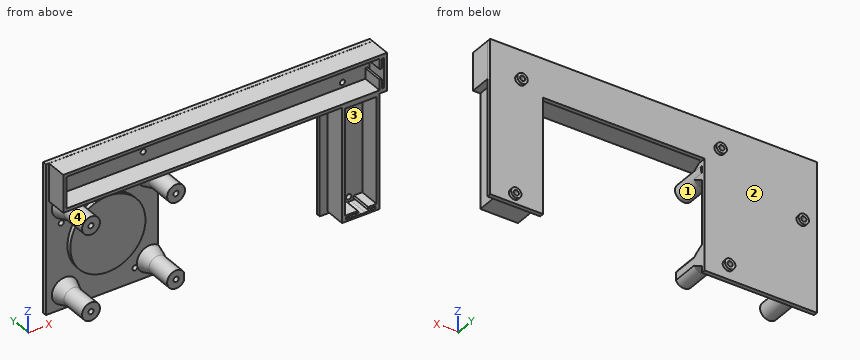
from build123d import *

# Parameters (mm, degrees)
SKETCH1_W                 = 25.299499494
SKETCH1_H                 = 55.159009877
SKETCH1_R                 = 1.241657959
SKETCH1_R_2               = 1.244649804
SKETCH1_R_3               = 1.243452392
SKETCH1_W_2               = 53.713568487
SKETCH1_H_2               = 52.951897156
SKETCH1_R_4               = 1.244762628
SKETCH1_R_5               = 1.240228495
BOSS_EXTRUDE1_DEPTH       = 2
SKETCH2_R                 = 2.521764251
SKETCH2_R_2               = 1.240228495
SKETCH2_R_3               = 2.471513498
SKETCH2_R_4               = 1.244762628
SKETCH2_R_5               = 2.485581318
SKETCH2_R_6               = 1.244649804
SKETCH2_R_7               = 2.50000008
SKETCH2_R_8               = 1.232345201
SKETCH2_R_9               = 2.472424153
SKETCH2_R_10              = 1.241657959
BOSS_EXTRUDE2_DEPTH       = 1.5
BOSS_EXTRUDE3_OUTLINE_R   = 4.264975471
BOSS_EXTRUDE3_OUTLINE_R_2 = 1.25
BOSS_EXTRUDE3_OUTLINE_R_3 = 4.293360572
BOSS_EXTRUDE3_DEPTH       = 18.2
BOSS_EXTRUDE4_OUTLINE_W   = 148.81215391
BOSS_EXTRUDE4_OUTLINE_H   = 14.000040224
BOSS_EXTRUDE4_DEPTH       = 10
SKETCH7_W                 = 18.030681689
SKETCH7_H                 = 1.47954917
BOSS_EXTRUDE5_DEPTH       = 10
SKETCH8_R                 = 2.5
SKETCH8_W                 = 14.030681689
SKETCH8_H                 = 1
CUT_EXTRUDE1_DEPTH        = 16.42
SKETCH9_W                 = 2
SKETCH9_H                 = 18.000040224
BOSS_EXTRUDE6_DEPTH       = 10
SKETCH10_W                = 1
SKETCH10_H                = 14.000040224
SKETCH10_W_2              = 1.5
SKETCH10_H_2              = 5
CUT_EXTRUDE2_DEPTH        = 10
CHAMFER1_SIZE             = 2
CHAMFER1_SIZE_2           = 5.494954839
SKETCH12_W                = 15.030681689
SKETCH12_H                = 50.706334577
SKETCH12_W_2              = 14.030681689
SKETCH12_H_2              = 49.706334577
SKETCH12_W_3              = 149.81215391
SKETCH12_H_3              = 15.000040224
SKETCH12_W_4              = 148.81215391
SKETCH12_H_4              = 14.000040224
CUT_EXTRUDE3_DEPTH        = 16.42
SKETCH13_R                = 17.983803221
BOSS_EXTRUDE7_DEPTH       = 2


# Read off the part's stored shape, not the designer's step: Boss-Extrude3, Boss-Extrude4
with BuildPart() as part:
    # Sketch1 → Boss-Extrude1 (new body)
    # profile 1 of 3: a face of its own
    with BuildSketch(Plane(origin=(0, 0, 0), x_dir=(1, 0, 0), z_dir=(0, 1, 0))):
        with Locations((-12.099843009, -21.166171701)):
            Rectangle(SKETCH1_W, SKETCH1_H)
        with Locations(Location((-10.884458073, 2.271979315, 0), (0, 0, 270))):
            Circle(SKETCH1_R, mode=Mode.SUBTRACT)
    # profile 2 of 3: a face of its own
    with BuildSketch(Plane(origin=(0, 0, 0), x_dir=(1, 0, 0), z_dir=(0, 1, 0))):
        Polygon((0.549906738, -67.187297417), (0.549906738, -48.745676639), (-24.749592756, -48.745676639), (-102.011751733, -48.745676639), (-155.72532022, -48.745676639), (-155.72532022, -67.187297417), align=None)
        with Locations(Location((-109.139310681, -55.741320352, 0), (0, 0, 270))):
            Circle(SKETCH1_R_2, mode=Mode.SUBTRACT)
        with Locations(Location((-13.892677204, -53.014877456, 0), (0, 0, 270))):
            Circle(SKETCH1_R_3, mode=Mode.SUBTRACT)
    # profile 3 of 3: a face of its own
    with BuildSketch(Plane(origin=(0, 0, 0), x_dir=(1, 0, 0), z_dir=(0, 1, 0))):
        with Locations((-128.868535977, -22.269728061)):
            Rectangle(SKETCH1_W_2, SKETCH1_H_2)
        with Locations(Location((-148.388511799, -36.727074265, 0), (0, 0, 270))):
            Circle(SKETCH1_R_4, mode=Mode.SUBTRACT)
        with Locations(Location((-113.148248588, -2.237044718, 0), (0, 0, 270))):
            Circle(SKETCH1_R_5, mode=Mode.SUBTRACT)
    extrude(amount=BOSS_EXTRUDE1_DEPTH)

    # Sketch2 → Boss-Extrude2 (add)
    # profile 1 of 5: a face of its own
    with BuildSketch(Plane(origin=(0, 2, 0), x_dir=(1, 0, 0), z_dir=(0, 1, 0))):
        with Locations(Location((-113.148248588, -2.237044718, 0), (0, 0, 270))):
            Circle(SKETCH2_R)
        with Locations(Location((-113.148248588, -2.237044718, 0), (0, 0, 270))):
            Circle(SKETCH2_R_2, mode=Mode.SUBTRACT)
    # profile 2 of 5: a face of its own
    with BuildSketch(Plane(origin=(0, 2, 0), x_dir=(1, 0, 0), z_dir=(0, 1, 0))):
        with Locations(Location((-148.388511799, -36.727074265, 0), (0, 0, 270))):
            Circle(SKETCH2_R_3)
        with Locations(Location((-148.388511799, -36.727074265, 0), (0, 0, 270))):
            Circle(SKETCH2_R_4, mode=Mode.SUBTRACT)
    # profile 3 of 5: a face of its own
    with BuildSketch(Plane(origin=(0, 2, 0), x_dir=(1, 0, 0), z_dir=(0, 1, 0))):
        with Locations(Location((-109.139310681, -55.741320352, 0), (0, 0, 270))):
            Circle(SKETCH2_R_5)
        with Locations(Location((-109.139310681, -55.741320352, 0), (0, 0, 270))):
            Circle(SKETCH2_R_6, mode=Mode.SUBTRACT)
    # profile 4 of 5: a face of its own
    with BuildSketch(Plane(origin=(0, 2, 0), x_dir=(1, 0, 0), z_dir=(0, 1, 0))):
        with Locations(Location((-13.886720738, -53.00550248, 0), (0, 0, 270))):
            Circle(SKETCH2_R_7)
        with Locations(Location((-13.886720738, -53.00550248, 0), (0, 0, 57.569834669))):
            Circle(SKETCH2_R_8, mode=Mode.SUBTRACT)
    # profile 5 of 5: a face of its own
    with BuildSketch(Plane(origin=(0, 2, 0), x_dir=(1, 0, 0), z_dir=(0, 1, 0))):
        with Locations(Location((-10.884458073, 2.271979315, 0), (0, 0, 270))):
            Circle(SKETCH2_R_9)
        with Locations(Location((-10.884458073, 2.271979315, 0), (0, 0, 270))):
            Circle(SKETCH2_R_10, mode=Mode.SUBTRACT)
    extrude(amount=BOSS_EXTRUDE2_DEPTH)

    # Boss-Extrude3 outline → Boss-Extrude3 (add)
    # profile 1 of 4: a face of its own
    with BuildSketch(Plane.XZ):
        with Locations((-105.874082677, 44.738348581)):
            Circle(BOSS_EXTRUDE3_OUTLINE_R)
        with Locations((-105.874082677, 44.738348581)):
            Circle(BOSS_EXTRUDE3_OUTLINE_R_2, mode=Mode.SUBTRACT)
    # profile 2 of 4: a face of its own
    with BuildSketch(Plane.XZ):
        with BuildLine():
            ThreePointArc((-102.011751733, 5.914823562), (-110.167443249, 4.039898313), (-102.011751733, 2.164973064))
            Line((-102.011751733, 2.164973064), (-102.011751733, 5.914823562))
        make_face()
        with Locations((-105.874082677, 4.039898313)):
            Circle(BOSS_EXTRUDE3_OUTLINE_R_2, mode=Mode.SUBTRACT)
    # profile 3 of 4: a face of its own
    with BuildSketch(Plane.XZ):
        with Locations((-146.574082677, 4.039898313)):
            Circle(BOSS_EXTRUDE3_OUTLINE_R_3)
        with Locations((-146.574082677, 4.039898313)):
            Circle(BOSS_EXTRUDE3_OUTLINE_R_2, mode=Mode.SUBTRACT)
    # profile 4 of 4: a face of its own
    with BuildSketch(Plane.XZ):
        with Locations((-146.574082677, 44.738348581)):
            Circle(BOSS_EXTRUDE3_OUTLINE_R)
        with Locations((-146.574082677, 44.738348581)):
            Circle(BOSS_EXTRUDE3_OUTLINE_R_2, mode=Mode.SUBTRACT)
    extrude(amount=BOSS_EXTRUDE3_DEPTH)

    # Boss-Extrude4 outline → Boss-Extrude4 (add)
    with BuildSketch(Plane.XZ):
        Polygon((-2.890953027, -4.07972047), (-2.890953027, 49.144078772), (-1.415765517, 49.144078772), (-1.415765517, 67.144118996), (-154.227919427, 67.144118996), (-154.227919427, 49.144078772), (-20.921634716, 49.144078772), (-20.921634716, -4.07972047), align=None)
        with BuildLine():
            ThreePointArc((-9.657775138, -2.07972047), (-10.884458073, -3.513637274), (-12.111141008, -2.07972047))
            Line((-12.111141008, -2.07972047), (-18.921634716, -2.07972047))
            Line((-18.921634716, -2.07972047), (-18.921634716, 47.626614107))
            Line((-18.921634716, 47.626614107), (-4.890953027, 47.626614107))
            Line((-4.890953027, 47.626614107), (-4.890953027, -2.07972047))
            Line((-4.890953027, -2.07972047), (-9.657775138, -2.07972047))
        make_face(mode=Mode.SUBTRACT)
        with Locations((-77.821842472, 58.144098884)):
            Rectangle(BOSS_EXTRUDE4_OUTLINE_W, BOSS_EXTRUDE4_OUTLINE_H, mode=Mode.SUBTRACT)
    extrude(amount=BOSS_EXTRUDE4_DEPTH)

    # Sketch7 → Boss-Extrude5 (add)
    with BuildSketch(Plane.XZ):
        with Locations((-11.906293872, -4.819495055)):
            Rectangle(SKETCH7_W, SKETCH7_H)
    extrude(amount=BOSS_EXTRUDE5_DEPTH)

    # Sketch8 → Cut-Extrude1 (cut)
    with BuildSketch(Plane.XZ):
        with Locations((-10.884458073, -2.271979315)):
            Circle(SKETCH8_R)
        with Locations((-11.906293872, -4.07972047)):
            Rectangle(SKETCH8_W, SKETCH8_H)
    extrude(amount=CUT_EXTRUDE1_DEPTH, mode=Mode.SUBTRACT)

    # Sketch9 → Boss-Extrude6 (add)
    with BuildSketch(Plane.XZ):
        with Locations((-0.415765517, 58.144098884)):
            Rectangle(SKETCH9_W, SKETCH9_H)
    extrude(amount=BOSS_EXTRUDE6_DEPTH)

    # Sketch10 → Cut-Extrude2 (cut)
    with BuildSketch(Plane.XZ.offset(10)):
        with Locations((-1.415765517, 58.144098884)):
            Rectangle(SKETCH10_W, SKETCH10_H)
        with Locations((-2.665765517, 58.144118996)):
            Rectangle(SKETCH10_W_2, SKETCH10_H_2)
    extrude(amount=-CUT_EXTRUDE2_DEPTH, mode=Mode.SUBTRACT)

    # Chamfer1
    # the kernel refuses this chamfer: 5.494954839, 2 mm, written as the material it adds along each edge
    with BuildSketch(Plane(origin=(-105.874082677, 0, 44.738348581), x_dir=(0.9999950652018582, 0, 0.0031415874859127522), z_dir=(0.0031415874859127522, 0, -0.9999950652018582))) as chamfer1_piece_1_section:
        Polygon((4.264975471 + CHAMFER1_SIZE, 0), (4.264975471, CHAMFER1_SIZE_2), (4.264975471, 0), align=None)
    chamfer1_piece_1 = revolve(axis=Axis((-105.874082677, 0, 44.738348581), (0, -1, 0)), revolution_arc=359.64, mode=Mode.PRIVATE)
    chamfer1_piece_1 = split(chamfer1_piece_1, bisect_by=Plane(origin=(-102.011751733, -2.257712416, 48.069640288), z_dir=(-1, 0, 0)), keep=Keep.TOP, mode=Mode.PRIVATE)
    add(chamfer1_piece_1)
    with BuildSketch(Plane(origin=(-105.874082677, 0, 44.738348581), x_dir=(0.9999950652018582, 0, 0.0031415874859127522), z_dir=(0.0031415874859127522, 0, -0.9999950652018582))) as chamfer1_piece_2_section:
        Polygon((4.264975471 + CHAMFER1_SIZE, 0), (4.264975471, CHAMFER1_SIZE_2), (4.264975471, 0), align=None)
    chamfer1_piece_2 = revolve(axis=Axis((-105.874082677, 0, 44.738348581), (0, -1, 0)), revolution_arc=359.64, mode=Mode.PRIVATE)
    chamfer1_piece_2 = split(chamfer1_piece_2, bisect_by=Plane(origin=(-101.74069423, -0.533251507, 48.745676639), z_dir=(0, 0, 1)), keep=Keep.TOP, mode=Mode.PRIVATE)
    add(chamfer1_piece_2)
    with BuildSketch(Plane(origin=(-105.874082676, 0, 4.039898313), x_dir=(0.9999950652018581, 0, 0.0031415874858793983), z_dir=(0.0031415874858793983, 0, -0.9999950652018581))) as chamfer1_piece_3_section:
        Polygon((4.293360573 + CHAMFER1_SIZE, 0), (4.293360573, CHAMFER1_SIZE_2), (4.293360573, 0), align=None)
    chamfer1_piece_3 = revolve(axis=Axis((-105.874082676, 0, 4.039898313), (0, -1, 0)), revolution_arc=359.64, mode=Mode.PRIVATE)
    chamfer1_piece_3 = split(chamfer1_piece_3, bisect_by=Plane(origin=(-102.011751733, -2.729942782, 4.039898313), z_dir=(-1, 0, 0)), keep=Keep.TOP, mode=Mode.PRIVATE)
    chamfer1_piece_3 = chamfer1_piece_3 - Plane(origin=(-113.148248588, -2.729942782, 2.237044718), x_dir=(0, 0, 1), z_dir=(0, -1, 0)) * Cylinder(1.240228495, 26, mode=Mode.PRIVATE)
    add(chamfer1_piece_3)
    with BuildSketch(Plane(origin=(-146.574082677, 0, 4.039898313), x_dir=(1, 0, 0), z_dir=(0, 0, -1))) as chamfer1_piece_4:
        Polygon((4.293360572 + CHAMFER1_SIZE, 0), (4.293360572, CHAMFER1_SIZE_2), (4.293360572, 0), align=None)
    revolve(axis=Axis((-146.574082677, 0, 4.039898313), (0, -1, 0)))
    with BuildSketch(Plane(origin=(-146.574082677, 0, 44.738348581), x_dir=(1, 0, 0), z_dir=(0, 0, -1))) as chamfer1_piece_5:
        Polygon((4.264975471 + CHAMFER1_SIZE, 0), (4.264975471, CHAMFER1_SIZE_2), (4.264975471, 0), align=None)
    revolve(axis=Axis((-146.574082677, 0, 44.738348581), (0, -1, 0)))

    # Sketch12 → Cut-Extrude3 (cut)
    # profile 1 of 2: a face of its own
    with BuildSketch(Plane.XZ):
        with Locations((-11.906293872, 22.773446819)):
            Rectangle(SKETCH12_W, SKETCH12_H)
        with Locations((-11.906293872, 22.773446819)):
            Rectangle(SKETCH12_W_2, SKETCH12_H_2, mode=Mode.SUBTRACT)
    # profile 2 of 2: a face of its own
    with BuildSketch(Plane.XZ):
        with Locations((-77.821842472, 58.144098884)):
            Rectangle(SKETCH12_W_3, SKETCH12_H_3)
        with Locations((-77.821842472, 58.144098884)):
            Rectangle(SKETCH12_W_4, SKETCH12_H_4, mode=Mode.SUBTRACT)
    extrude(amount=CUT_EXTRUDE3_DEPTH, mode=Mode.SUBTRACT)

    # Sketch13 → Boss-Extrude7 (add)
    with BuildSketch(Plane(origin=(0, 0, 0), x_dir=(-1, 0, 0), z_dir=(0, -1, 0))):
        with Locations(Location((127.431607473, -24.759221512, 0), (0, 0, 270))):
            Circle(SKETCH13_R)
    extrude(amount=BOSS_EXTRUDE7_DEPTH)


solid = part.part
Source: CAD feature listing. Evaluate the final solid. Frame: model axes, mm. Face numbers are marked on the shaded views. A direction names the side the tool comes from. Round coordinates to 2 decimals unless told otherwise and drop trailing zeros. Loops run counter-clockwise (first coordinate to the right, second up) from the corner with the lowest first, then second, coordinate; pieces in that order, holes last.
Q1. Section A-A, the plane y = -11.75. Return loops of the section in (x, z).
Q2. First-contact query: P1, Ø1.1, axis at y = -6.5, z = -4, coming from the +X side; P2, Ø3, axis at x = -11, y = -4, coming from the -Z side; P3, Ø5, axis at x = -107.5, y = -1.5, coming from the -Z side; P4, Ø1.5, axis at x = -13.89, z = 53.01, coming from the +Y side. Flat tips, straight axial feed; report the tip coordinate or a pass-through.
Q3. Section D-D, the plane x = -118. Return loops of the section in (y, z), plus the area to 3 significant figures.
Q4. Mould query, pull axis X, two halves, no side actions, for the marked faces 3 and 4. Classes: pulls with the +X half, pulls with the -X half, needs draft (parallel to the pull), parting line crosses it, or undercut.
Q5. Access query for the marked faces 1 and 2. Directions: +Z, -Z, +X, -X, +Y, -Y. A direction counts if a zero-diameter tool reaches every point of the face in a straight line with its end or side. Return the directions, or none.
Q6. Section C-C, the plane x = -38. Return loops of the section in (y, z), plus the area to 3 significant figures.
Q7. Section B-B, the plane z = 14. Return loops of the section in (x, y), plus the area to 3 significant figures.
Q8. Ray query, line 1 (Z direction, x = -7, y = -4); line 2 (Z direction, x = -10, y = -7.75); line 3 (X direction, y = -9.5, z = 61). Return the intervals inside material, ascending.
Solutions:
1. outline: circle Ø8.59 at (-146.57, 4.04); circle Ø8.53 at (-146.57, 44.74); circle Ø8.53 at (-105.87, 44.74); (-102.01, 2.16) - (-102.01, 5.91) arc R4.29 ccw (long way) to start; hole circle Ø2.5 at (-146.57, 4.04); hole circle Ø2.5 at (-146.57, 44.74); hole circle Ø2.5 at (-105.87, 4.04); hole circle Ø2.5 at (-105.87, 44.74)
2. P1: stops at x = -2.89
2. P2: stops at z = -5.56
2. P3: stops at z = -4.21
2. P4: passes through
3. outline: (-10, 49.14) - (0, 49.14) - (0, 40.07) - (-2, 40.07) - (-2, 9.45) - (0, 9.45) - (0, -4.21) - (2, -4.21) - (2, 67.19) - (0, 67.19) - (0, 67.14) - (-10, 67.14) - (-10, 65.64) - (0, 65.64) - (0, 50.64) - (-10, 50.64) - close
3. area: 234 mm2
4. face 3: undercut
4. face 4: undercut
5. face 1: -Y
5. face 2: +Y
6. outline: (-10, 49.14) - (0, 49.14) - (0, 48.75) - (2, 48.75) - (2, 67.19) - (0, 67.19) - (0, 67.14) - (-10, 67.14) - (-10, 65.64) - (0, 65.64) - (0, 50.64) - (-10, 50.64) - close
6. area: 66.9 mm2
7. outline: (-155.73, 0) - (-141.84, 0) - (-141.84, -2) - (-113.02, -2) - (-113.02, 0) - (-102.01, 0) - (-102.01, 2) - (-155.73, 2) - close; (-24.75, 0) - (-20.92, 0) - (-20.92, -10) - (-19.42, -10) - (-19.42, 0) - (-4.39, 0) - (-4.39, -10) - (-2.89, -10) - (-2.89, 0) - (0.55, 0) - (0.55, 2) - (-24.75, 2) - close
7. area: 246 mm2
8. line 1: z = -5.56 to -4.58, -3.58 to -2.58, 48.13 to 50.64, 65.64 to 67.14
8. line 2: z = -5.56 to -4.61, 48.13 to 50.64, 65.64 to 67.14
8. line 3: x = -154.23 to -152.73, -2.92 to -1.92, -0.92 to 0.58
